Here's the drawing with two shaded views (mm, measured from the low corner). I have some questions. A direction names the side the tool comes from. Give positions to 0.01 mm unless a question says otherwise; leave off trailing zeros. Loops run counter-clockwise (first coordinate to the right, second up) from the corner with the lowest first, then second, coordinate; pieces in that order, holes last. Notation, with made-up numbers: (54.25, 83) -> (85.25, 83) arc R26 ccw to (85.25, 122) -> close; hole circle Ø8 at (-8, 35). An arc over 180 degrees is marked (long way). Answer in a Markdown table with one row per item. Add a question column.
Item 1: Which directions (+Z, -Z, +X, -X, +Y, -Y) give clear straight access to the entire face, cutting with the end or side of a thin tool? Please do the marked faces 1 and 2.
Item 2: If we section it at D-D (y = 11.5): Write out the boundary of the cut face in (x, z).
Item 3: If we section it at A-A (x = 25.4): Write out the boundary of the cut face in (y, z), then the cut area to 3 significant figures.
Item 4: If we section it at C-C (z = 31): Write out the boundary of the cut face in (x, y).
Item 5: For P1, Ø10, axis at x = 28, z = 12, coming from the -Y side, with a flat end and sliding along its axis, tell me the tip position at first contact or that it passes through.
Item 6: If I drill on line 1 (Y direction, x = 52, z = 37); line 2 (Z direction, x = 25.4, y = 14); line 3 (Z direction, x = 25.4, y = 12), over which ranges is the centre line in solid material (lowest first)?
Item 7: If we section it at B-B (y = 19): Write out the boundary of the cut face in (x, z), then the cut area to 3 significant figures.
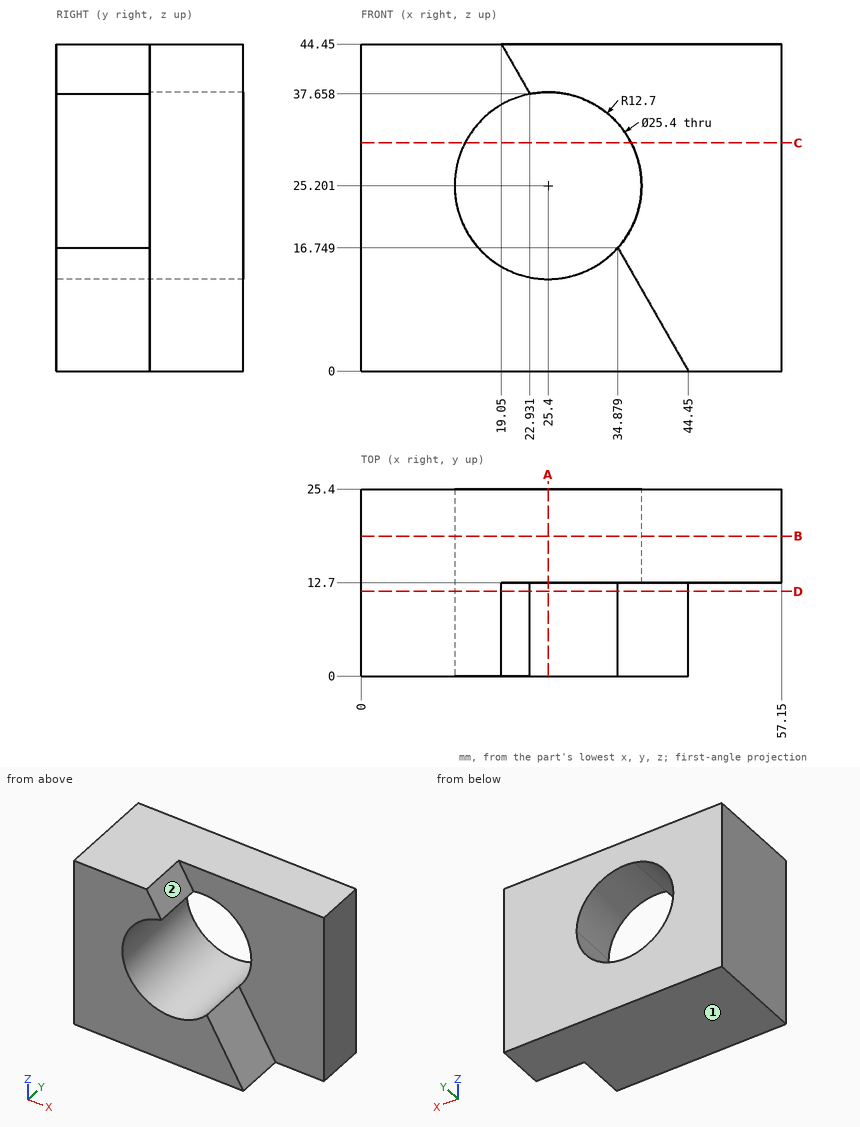
Recorded:
| question | item | result |
|---|---|---|
| 1 | face 1 | -Z, +X, -X, +Y, -Y |
| 1 | face 2 | +Z, +X, -Y |
| 2 | outline | (0, 0) -> (44.45, 0) -> (34.88, 16.75) arc R12.7 cw (long way) to (22.93, 37.66) -> (19.05, 44.45) -> (0, 44.45) -> close |
| 3 | outline | (0, 0) -> (25.4, 0) -> (25.4, 12.5) -> (0, 12.5) -> close; (12.7, 37.9) -> (25.4, 37.9) -> (25.4, 44.45) -> (12.7, 44.45) -> close |
| 3 | area | 401 mm^2 |
| 4 | outline | (0, 0) -> (14.1, 0) -> (14.1, 25.4) -> (0, 25.4) -> close; (36.7, 12.7) -> (57.15, 12.7) -> (57.15, 25.4) -> (36.7, 25.4) -> close |
| 5 | P1 | stops at y = 0 |
| 6 | line 1 | y = 12.7 to 25.4 |
| 6 | line 2 | z = 0 to 12.5, 37.9 to 44.45 |
| 6 | line 3 | z = 0 to 12.5 |
| 7 | outline | (0, 0) -> (57.15, 0) -> (57.15, 44.45) -> (0, 44.45) -> close; hole circle Ø25.4 at (25.4, 25.2) |
| 7 | area | 2,030 mm^2 |
